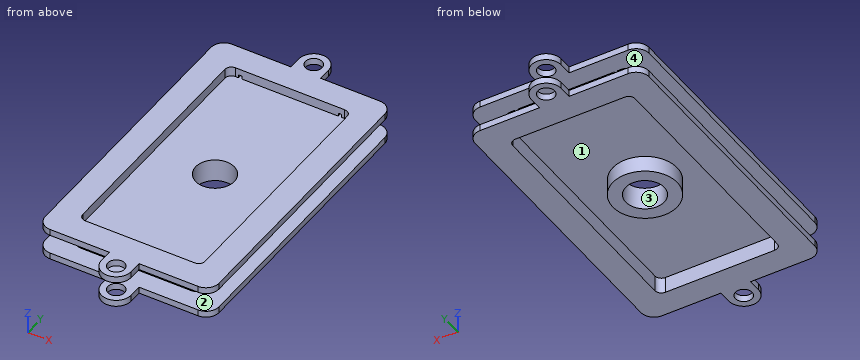
```python
from build123d import *

# Parameters (mm, degrees)
F1_DEPTH  = 1
F3_DEPTH  = 3
F4_DEPTH  = 1.001
F6_DEPTH  = 1
F7_R      = 1.3
F8_DEPTH  = 1
F10_W     = 19
F10_H     = 38
F11_DEPTH = 1
F12_R     = 3
F13_DEPTH = 25
F14_R     = 5
F14_R_2   = 3
F15_DEPTH = 2.5
F16_W     = 0.5
F16_H     = 0.5
F17_DEPTH = 5


# Not quite as in the source:
# - a pattern or mirror of a feature is missing from the dataset's text; its kind, count and spacing are read off the source's solid


with BuildPart() as f1:
    # F0 (on Top) → F1 (new body)
    with BuildSketch(Plane.XY):
        with BuildLine():
            ThreePointArc((13.5, 21), (12.9142135624, 22.4142135624), (11.5, 23))
            Line((11.5, 23), (-11.5, 23))
            ThreePointArc((-11.5, 23), (-12.9142135624, 22.4142135624), (-13.5, 21))
            Line((-13.5, 21), (-13.5, -21))
            ThreePointArc((-13.5, -21), (-12.9142135624, -22.4142135624), (-11.5, -23))
            Line((-11.5, -23), (11.5, -23))
            ThreePointArc((11.5, -23), (12.9142135624, -22.4142135624), (13.5, -21))
            Line((13.5, -21), (13.5, 21))
        make_face()
    extrude(amount=F1_DEPTH)

    # F2 (on face) → F3 (join)
    with BuildSketch(Plane.XY.offset(1)):
        with BuildLine():
            ThreePointArc((10.5, 18), (9.9142135624, 19.4142135624), (8.5, 20))
            Line((8.5, 20), (-8.5, 20))
            ThreePointArc((-8.5, 20), (-9.9142135624, 19.4142135624), (-10.5, 18))
            Line((-10.5, 18), (-10.5, -18))
            ThreePointArc((-10.5, -18), (-9.9142135624, -19.4142135624), (-8.5, -20))
            Line((-8.5, -20), (8.5, -20))
            ThreePointArc((8.5, -20), (9.9142135624, -19.4142135624), (10.5, -18))
            Line((10.5, -18), (10.5, 18))
        make_face()
        with BuildLine():
            ThreePointArc((8.5, 19), (9.2071067812, 18.7071067812), (9.5, 18))
            Line((9.5, 18), (9.5, -18))
            ThreePointArc((9.5, -18), (9.2071067812, -18.7071067812), (8.5, -19))
            Line((8.5, -19), (-8.5, -19))
            ThreePointArc((-8.5, -19), (-9.2071067812, -18.7071067812), (-9.5, -18))
            Line((-9.5, -18), (-9.5, 18))
            ThreePointArc((-9.5, 18), (-9.2071067812, 18.7071067812), (-8.5, 19))
            Line((-8.5, 19), (8.5, 19))
        make_face(mode=Mode.SUBTRACT)
    extrude(amount=F3_DEPTH)

    # F4 (cut, through all): a face of the model
    f4_faces = [f1.faces().sort_by_distance(p)[0] for p in [
        (0, 0, 1),
    ]]
    extrude(f4_faces, amount=-F4_DEPTH, mode=Mode.SUBTRACT)

    # F5 (on face) → F6 (join)
    with BuildSketch(Plane.XY.offset(4)):
        with BuildLine():
            Line((13.5, -21), (13.5, 21))
            ThreePointArc((13.5, 21), (12.9142135624, 22.4142135624), (11.5, 23))
            Line((11.5, 23), (-11.5, 23))
            ThreePointArc((-11.5, 23), (-12.9142135624, 22.4142135624), (-13.5, 21))
            Line((-13.5, 21), (-13.5, -21))
            ThreePointArc((-13.5, -21), (-12.9142135624, -22.4142135624), (-11.5, -23))
            Line((-11.5, -23), (11.5, -23))
            ThreePointArc((11.5, -23), (12.9142135624, -22.4142135624), (13.5, -21))
        make_face()
        with BuildLine():
            ThreePointArc((8.5, 19), (9.2071067812, 18.7071067812), (9.5, 18))
            Line((9.5, 18), (9.5, -18))
            ThreePointArc((9.5, -18), (9.2071067812, -18.7071067812), (8.5, -19))
            Line((8.5, -19), (-8.5, -19))
            ThreePointArc((-8.5, -19), (-9.2071067812, -18.7071067812), (-9.5, -18))
            Line((-9.5, -18), (-9.5, 18))
            ThreePointArc((-9.5, 18), (-9.2071067812, 18.7071067812), (-8.5, 19))
            Line((-8.5, 19), (8.5, 19))
        make_face(mode=Mode.SUBTRACT)
    extrude(amount=F6_DEPTH)

    # F7 (on Top) → F8 (join)
    with BuildSketch(Plane.XY):
        with BuildLine():
            Line((2.3, 23), (2.3, 25))
            ThreePointArc((2.3, 25), (0, 27.3), (-2.3, 25))
            Line((-2.3, 25), (-2.3, 23))
            Line((-2.3, 23), (2.3, 23))
        make_face()
        with Locations((0, 25)):
            Circle(F7_R, mode=Mode.SUBTRACT)
        with BuildLine():
            ThreePointArc((-2.3, -25), (0, -27.3), (2.3, -25))
            Line((2.3, -25), (2.3, -23))
            Line((2.3, -23), (-2.3, -23))
            Line((-2.3, -23), (-2.3, -25))
        make_face()
        with Locations((0, -25)):
            Circle(F7_R, mode=Mode.SUBTRACT)
    f8 = extrude(amount=F8_DEPTH)

    # F8_copies: F8 across plane
    add(f8.mirror(Plane.XY.offset(2.5)))

    # F10 (on mid) → F11 (join)
    with BuildSketch(Plane(origin=(0, 0, 2.5), x_dir=(1, 0, 0), z_dir=(0, 0, -1))):
        Rectangle(F10_W, F10_H)
    extrude(amount=-F11_DEPTH)

    # F12 (on face) → F13 (cut)
    with BuildSketch(Plane.XY.offset(3.5)):
        Circle(F12_R)
    extrude(amount=-F13_DEPTH, mode=Mode.SUBTRACT)

    # F14 (on face) → F15 (join, through all)
    with BuildSketch(Plane(origin=(0, 0, 2.5), x_dir=(1, 0, 0), z_dir=(0, 0, -1))):
        Circle(F14_R)
        Circle(F14_R_2, mode=Mode.SUBTRACT)
    extrude(amount=F15_DEPTH)

    # F16 (on face) → F17 (cut)
    with BuildSketch(Plane(origin=(0, 20, 0), x_dir=(-1, 0, 0), z_dir=(0, 1, 0))):
        with Locations((-7.75, 3.75)):
            Rectangle(F16_W, F16_H)
        with Locations((7.75, 3.75)):
            Rectangle(F16_W, F16_H)
    extrude(amount=-F17_DEPTH, mode=Mode.SUBTRACT)


solid = f1.part
```
Could you check a few things on this model? Use its own coordinates, in mm. Face numbers are marked on the shaded views. A direction names the side the tool comes from. Round coordinates to 2 decimals unless told otherwise and drop trailing zeros. Loops run counter-clockwise (first coordinate to the right, second up) from the corner with the lowest first, then second, coordinate; pieces in that order, holes last. Notation, with made-up numbers: (75.5, 45) - (105.5, 45) arc R26 ccw to (105.5, 70) - close; hole circle Ø4 at (82.25, 61). An arc over 180 degrees is marked (long way). Answer as CSV lines item,"result".
1. I want a section at A-A on y = 0. List the corners of the cut face in (x, z) for me.
Filled in:
outline,"(-13.5, 0) - (-9.5, 0) - (-9.5, 2.5) - (-5, 2.5) - (-5, 0) - (-3, 0) - (-3, 3.5) - (-9.5, 3.5) - (-9.5, 5) - (-13.5, 5) - (-13.5, 4) - (-10.5, 4) - (-10.5, 1) - (-13.5, 1) - close; (3, 0) - (5, 0) - (5, 2.5) - (9.5, 2.5) - (9.5, 0) - (13.5, 0) - (13.5, 1) - (10.5, 1) - (10.5, 4) - (13.5, 4) - (13.5, 5) - (9.5, 5) - (9.5, 3.5) - (3, 3.5) - close"
2. I want a section at D-D on x = 0. Count the separate pieces of the cut face and the enclosed holes in it, then the cut area to 3 significant figures.
Filled in:
separate pieces,"6"
enclosed holes,"0"
area,"70.8 mm^2"
3. I want a section at C-C on x = 7. List the corners of the cut face in (y, z) for me, then the cut area to 3 significant figures.
Filled in:
outline,"(-23, 0) - (-19, 0) - (-19, 2.5) - (19, 2.5) - (19, 0) - (23, 0) - (23, 1) - (20, 1) - (20, 4) - (23, 4) - (23, 5) - (19, 5) - (19, 3.5) - (-19, 3.5) - (-19, 5) - (-23, 5) - (-23, 4) - (-20, 4) - (-20, 1) - (-23, 1) - close"
area,"60.0 mm^2"
4. On a 3-axis mill with a long thin cutter (end or side, diameter ignored), from which of +Z, -Z, +X, -X, +Y, -Y can I reach the whole of each face in a straight line? I mean the marked faces 3 and 4. Say none if no direction works.
Filled in:
face 3,"+Z, -Z"
face 4,"none"
5. Please list where these lines run through material, in increasing order: line 1 along Y through (x, z) = (0, 0.6); line 2 along Y through (x, z) = (0, 4.45); line 3 along Y through (x, z) = (5, 4.7). Write a range as [from, to].
Filled in:
line 1,"y = [-27.3, -26.3], [-23.7, -19], [-5, -3], [3, 5], [19, 23.7], [26.3, 27.3]"
line 2,"y = [-27.3, -26.3], [-23.7, -19], [19, 23.7], [26.3, 27.3]"
line 3,"y = [-23, -19], [19, 23]"
6. For pin 1 Ø1.5 at (x, y) = (7, -16) entering from -Z; pin 2 Ø0.5 at (x, z) = (-7, 4.5) entering from -Y; pin 3 Ø2 at (x, y) = (0, -25) entering from -Z; pin 4 Ø2 at (x, z) = (-3, 2.5) entering from -Y, each with a flat end and sliding along its axis, tell me the tip position at first contact or that it passes through.
Filled in:
pin 1,"stops at z = 2.5"
pin 2,"stops at y = -23"
pin 3,"passes through"
pin 4,"stops at y = -20"
7. I want a section at B-B on y = 13.5. List the corners of the cut face in (x, z) for me, then the cut area to 3 significant figures.
Filled in:
outline,"(-13.5, 0) - (-9.5, 0) - (-9.5, 2.5) - (9.5, 2.5) - (9.5, 0) - (13.5, 0) - (13.5, 1) - (10.5, 1) - (10.5, 4) - (13.5, 4) - (13.5, 5) - (9.5, 5) - (9.5, 3.5) - (-9.5, 3.5) - (-9.5, 5) - (-13.5, 5) - (-13.5, 4) - (-10.5, 4) - (-10.5, 1) - (-13.5, 1) - close"
area,"41.0 mm^2"
8. We'd pull the mould along X, two halves only. Please class the marked faces 1 and 2: +X half, -X half, draft (parallel to the pull), parting line (faces both ways), or undercut.
Filled in:
face 1,"undercut"
face 2,"draft"
